Part model, mm, in its own coordinate system. Face numbers are marked on the shaded views. A direction names the side the tool comes from. Coordinates: 2 decimals unless noted, no trailing zeros. Write each loop counter-clockwise with the first axis right and the second up, starting at its lowest first coordinate (ties: lowest second). Pieces come first, ordered by that corner, then holes. Notation, with made-up numbers: (-7.5, 0) -> (22.5, 0) arc R9 cw to (22.5, 12) -> close; hole circle Ø6 at (78.5, 69). An arc over 180 degrees is marked (long way). Write item = value, one per line.
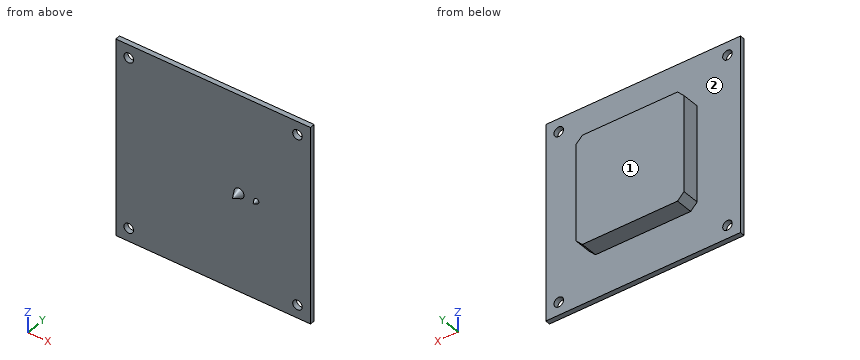
Autodesk Inventor part; units mm, degrees
ref_plane "Work Plane1" through (-12.5, 0, -22.5) normal (0, 0, 1) x (-1, 0, 0)
ref_plane "YZ Plane" through (0, 0, 0) normal (1, 0, 0) x (0, 1, 0)
ref_plane "XZ Plane" through (0, 0, 0) normal (0, 1, 0) x (-1, 0, 0)
sketch "Sketch1" plane through (0, 0, 0) normal (0, 1, 0) x (-1, 0, 0)
  line L0 (0, 0) -> (45, 0)
  line L1 (45, 0) -> (45, -45)
  line L2 (45, -45) -> (0, -45)
  line L3 (0, -45) -> (0, 0)
  dimension "d0" = 45
  dimension "d1" = 45
extrude "Extrusion1" add sketch "Sketch1" along normal blind 1.15
sketch "Sketch2" plane through (0, 1.15, 0) normal (0, 1, 0) x (1, 0, 0)
  line L0 (-45, 45) -> (-45, 0)
  line L1 (-45, 0) -> (-45, 3)
  line L2 (-45, 3) -> (-42, 3)
  line L3 (-45, 22.5) -> (-42, 22.5)
  line L4 (-45, 45) -> (-45, 42)
  line L5 (-45, 42) -> (-42, 42)
  line L6 (0, 45) -> (-45, 45)
  line L7 (-22.5, 45) -> (-22.5, 42.897)
  line L8 (0, 45) -> (0, 0)
  line L9 (0, 0) -> (0, 3)
  line L10 (0, 3) -> (-3, 3)
  line L11 (0, 22.5) -> (-3, 22.5)
  line L12 (0, 45) -> (0, 42)
  line L13 (0, 42) -> (-3, 42)
  dimension "d4" = 3
  dimension "d5" = 3
hole "Hole1" at (-42, 1.15, -3) at (-42, 1.15, -42) at (-3, 1.15, -42) at (-3, 1.15, -3) direction (0, -1, 0) diameter 2.2 end through all
sketch "Sketch3" plane through (0, 1.15, 0) normal (0, 1, 0) x (1, 0, 0)
  line L0 (-45, 0) -> (-45, 45)
  line L1 (0, 45) -> (0, 0)
  line L2 (-45, 45) -> (0, 45)
  line L3 (-35, 10) -> (-10, 10)
  line L4 (-10, 10) -> (-10, 35)
  line L5 (-10, 35) -> (-35, 35)
  line L6 (-35, 10) -> (-35, 35)
  dimension "d15" = 25
  dimension "d16" = 25
  dimension "d17" = 10
  dimension "d18" = 10
  dimension "d19" = 10
extrude "Extrusion2" add sketch "Sketch3" along normal blind 4
chamfer "Chamfer1" distance 1.5 angle 45 4 edges at (-10, 3.15, -35) (-35, 3.15, -35) (-10, 3.15, -10) (-35, 3.15, -10)
sketch "Sketch4" plane through (0, 0, 0) normal (0, -1, 0) x (1, 0, 0)
  line L0 (0, 0) -> (0, -45)
  line L1 (0, -22.5) -> (-12.5, -22.5)
  line L2 (-12.5, -22.5) -> (-16.5, -22.5)
  circle A0 centre (-12.5, -22.5) radius 0.5
  circle A1 centre (-16.5, -22.5) radius 0.5
  dimension "d25" = 12.5
  dimension "d26" = 4
  dimension "d27" = 1
ref_plane "Work Plane1" through (-12.5, 0, -22.5) normal (0, 0, 1) x (-1, 0, 0)
sketch "Sketch5" plane through (-12.5, 0, -22.5) normal (0, 0, 1) x (-1, 0, 0)
  line L0 (0, 0) -> (4, 0)
  line L1 (-12.5, 0) -> (0, 0)
  line L2 (4, 0) -> (4, 2)
  line L3 (4, 0) -> (5.15, 0)
  line L4 (4, 2) -> (5.15, 0)
  line L5 (0, 0) -> (0.575, 0)
  point P0 (-12.5, 0)
  dimension "d31" = 2
  dimension "d33" = 1.15
revolve "Revolution1" add sketch "Sketch5" angle 360 about axis through (-16.5, 0, -22.5) along (0, -1, 0)
sketch "Sketch6" plane through (-12.5, 0, -22.5) normal (0, 0, 1) x (-1, 0, 0)
  line L0 (0, 0) -> (0, 1)
  line L1 (0, 0) -> (0.575, 0)
  line L2 (0, 1) -> (0.575, 0)
  point P0 (-12.5, 0)
  dimension "d36" = 1
  dimension "d37" = 0.575
revolve "Revolution2" add sketch "Sketch6" angle 360 about axis through (-12.5, 0, -22.5) along (0, -1, 0)
properties part number "Patch_Antenna_V1"
Q1. Saw through at C-C on y = 3.25. Give the cut face in (x, z), and give its area (4 significant figures).
Model answer:
outline = (-35, -33.5) -> (-33.5, -35) -> (-11.5, -35) -> (-10, -33.5) -> (-10, -11.5) -> (-11.5, -10) -> (-33.5, -10) -> (-35, -11.5) -> close
area = 620.5 mm²
Q2. Pin check, flat tips, straight feed: pin 1 (1.2 mm diameter, centred on x = -19, y = 3, fed in from -Z); pin 2 (3.5 mm diameter, centred on x = -3, z = -3, fed in from +Y); pin 3 (3.5 mm diameter, centred on x = -3, z = -42, fed in from -Y); pin 4 (1.8 mm diameter, centred on x = -42, z = -3, fed in from +Y). Stop position of each tip, or through.
Model answer:
pin_1 = -35
pin_2 = 1.15
pin_3 = 0
pin_4 = through
Q3. Saw through at A-A on z = -3. Give the cut face in (x, y).
Model answer:
outline = (-45, 0) -> (-43.1, 0) -> (-43.1, 1.15) -> (-45, 1.15) -> close; (-40.9, 0) -> (-4.1, 0) -> (-4.1, 1.15) -> (-40.9, 1.15) -> close; (-1.9, 0) -> (0, 0) -> (0, 1.15) -> (-1.9, 1.15) -> close
Q4. Probe line 1 (X direction, y = 0.75, z = -3); line 2 (Y direction, x = -38.5, z = -36.5). List the from-to ranges inside material, lowest first. Write a range as from..to.
Model answer:
line_1 = -45..-43.1, -40.9..-4.1, -1.9..0
line_2 = 0..1.15
Q5. Which spindle directions (+Z, -Z, +X, -X, +Y, -Y) get a long thin tool onto all of the face, cutting with end or side? Do the marked faces 1 and 2. Say none if no direction does.
Model answer:
face_1 = +Z, -Z, +X, -X, +Y
face_2 = +Y
Q6. Saw through at B-B on x = -42. Give the cut face in (y, z).
Model answer:
outline = (0, -45) -> (1.15, -45) -> (1.15, -43.1) -> (0, -43.1) -> close; (0, -40.9) -> (1.15, -40.9) -> (1.15, -4.1) -> (0, -4.1) -> close; (0, -1.9) -> (1.15, -1.9) -> (1.15, 0) -> (0, 0) -> close
Q7. Saw through at D-D on x = -22. Give the cut face in (y, z), and give its area (3 significant figures).
Model answer:
outline = (0, -45) -> (1.15, -45) -> (1.15, -35) -> (5.15, -35) -> (5.15, -10) -> (1.15, -10) -> (1.15, 0) -> (0, 0) -> close
area = 152 mm²
